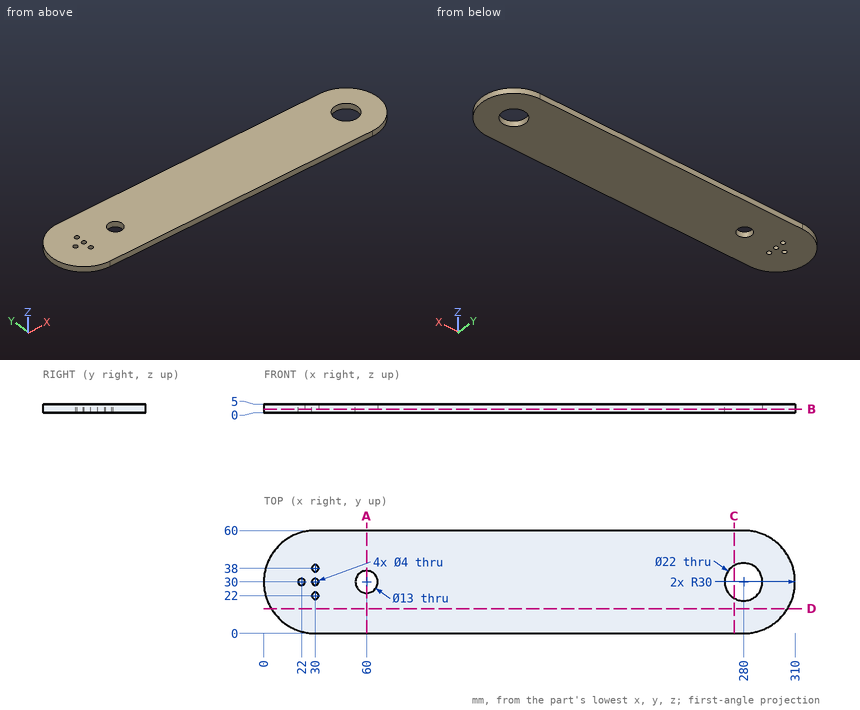
Study the drawing (mm; zero at the part's minimum x, y, z) and answer. Give positions to 0.01 mm unless a question says otherwise; leave off trailing zeros. Order: outer loops, then holes, each group sorted by start corner. A loop starts at its lowest first (then second) coordinate and runs counter-clockwise, first axis right, second up. Notation, with made-up numbers: (46.25, 14) - (103.25, 14) arc R20 cw to (103.25, 53) - close; hole circle Ø5 at (-16.5, 72). An arc over 180 degrees is marked (long way). Answer in a Markdown table with one row per item. Add a question column.
Q1. The part is cut by section D-D (y = 14.5). Determine the outline of the cut face in (x, z), then the cut area to 3 significant figures.
Q2. Find the intervals of material crossed by line 1 along Y through (x, z) = (30, 3.15); line 2 along Y through (x, z) = (280, 3.15); line 3 along X through (y, z) = (33.5, 2.4), in increasing order. Write a range as [from, to].
Q3. The part is cut by section B-B (z = 1.95). Determine the outline of the cut face in (x, y), then the cut area to 3 significant figures.
Q4. The part is cut by section C-C (x = 274.5). Determine the outline of the cut face in (y, z).
Q5. The part is cut by section A-A (x = 60). Determine the outline of the cut face in (y, z), then the cut area to 3 significant figures.
Determined:
| question | item | result |
|---|---|---|
| 1 | outline | (4.31, 0) - (305.69, 0) - (305.69, 5) - (4.31, 5) - close |
| 1 | area | 1,510 mm² |
| 2 | line 1 | y = [0, 20], [24, 28], [32, 36], [40, 60] |
| 2 | line 2 | y = [0, 19], [41, 60] |
| 2 | line 3 | x = [0.2, 54.52], [65.48, 269.57], [290.43, 309.8] |
| 3 | outline | (30, 0) - (280, 0) arc R30 ccw to (280, 60) - (30, 60) arc R30 ccw to start; hole circle Ø4 at (22, 30); hole circle Ø4 at (30, 22); hole circle Ø4 at (30, 30); hole circle Ø4 at (30, 38); hole circle Ø13 at (60, 30); hole circle Ø22 at (280, 30) |
| 3 | area | 17,300 mm² |
| 4 | outline | (0, 0) - (20.47, 0) - (20.47, 5) - (0, 5) - close; (39.53, 0) - (60, 0) - (60, 5) - (39.53, 5) - close |
| 5 | outline | (0, 0) - (23.5, 0) - (23.5, 5) - (0, 5) - close; (36.5, 0) - (60, 0) - (60, 5) - (36.5, 5) - close |
| 5 | area | 235 mm² |
